For this review, take the finished solid that the model builds, in its own axes (mm). Face numbers are marked on the shaded views. A direction names the side the tool comes from. Coordinates: 2 decimals unless noted, no trailing zeros. Loops run counter-clockwise (first coordinate to the right, second up) from the corner with the lowest first, then second, coordinate; pieces in that order, holes last. Notation, with made-up numbers: (85.5, 34.5) - (126.5, 34.5) arc R20 cw to (126.5, 61.5) - close; hole circle Ø9 at (23, 58.25). An arc over 180 degrees is marked (long way). Answer as a JSON object with one key per item and string values. Group by question number.
Item 1: To check wall thickness, follow line 1 (Y direction, x = 3, z = -38.5); line 2 (Z direction, x = 1.7, y = -1.3); line 3 (Z direction, x = 2.35, y = 0.3). State the ranges of each line that lie inside material, in increasing order.
Item 2: Tool access review of the marked faces 1, 2 and 3: name each direction out of +Z, -Z, +X, -X, +Y, -Y from which nothing blocks a thin tool from reaching the whole face with its end or side.
Item 3: We need section B-B (x = 2.25). Give the boundary of the cut face in (y, z), then the cut area to 3 significant figures.
Item 4: We need section A-A (y = 0). Give the boundary of the cut face in (x, z).
Item 5: We need section C-C (z = -38). Give the boundary of the cut face in (x, y).
Item 6: Clearance check with flat-ended pins moving along their axes: pin 1 (3 mm diameter, centred on y = 0, z = -38.5, fed in from -X); pin 2 (3 mm diameter, centred on y = -1, z = -3.5, fed in from +X); pin 3 (0.6 mm diameter, centred on x = 3.5, y = -0.5, fed in from +Z); pin 4 (0.6 mm diameter, centred on x = 0.5, y = -1, fed in from -Z). State where each tip first meets the part, or that it passes through.
Item 7: We need section D-D (x = 0.55). Give the boundary of the cut face in (y, z), then the cut area to 3 significant figures.
from build123d import *

# Parameters (mm, degrees)
SKETCH1_R           = 1.65
BOSS_EXTRUDE1_DEPTH = 3
SKETCH3_W           = 11
SKETCH3_H           = 6
CUT_EXTRUDE2_DEPTH  = 1.2
SKETCH4_R           = 1.65
BOSS_EXTRUDE2_DEPTH = 1.2


with BuildPart() as part:
    # Sketch1 → Boss-Extrude1 (new body)
    with BuildSketch(Plane(origin=(0, 0, 0), x_dir=(0, 0, -1), z_dir=(1, 0, 0))):
        with BuildLine():
            Line((0, 3), (38.5, 3))
            ThreePointArc((38.5, 3), (41.5, 0), (38.5, -3))
            Line((38.5, -3), (0, -3))
            ThreePointArc((0, -3), (-3, 0), (0, 3))
        make_face()
        Circle(SKETCH1_R, mode=Mode.SUBTRACT)
        with Locations((38.5, 0)):
            Circle(SKETCH1_R, mode=Mode.SUBTRACT)
    extrude(amount=BOSS_EXTRUDE1_DEPTH)

    # Sketch3 → Cut-Extrude2 (cut)
    with BuildSketch(Plane.ZY):
        with Locations((-36, 0)):
            Rectangle(SKETCH3_W, SKETCH3_H)
    extrude(amount=-CUT_EXTRUDE2_DEPTH, mode=Mode.SUBTRACT)

    # Sketch4 → Boss-Extrude2 (add)
    with BuildSketch(Plane(origin=(3, 0, 0), x_dir=(0, 0, -1), z_dir=(1, 0, 0))):
        with BuildLine():
            Line((38.5, 3), (21.5, 3))
            Line((21.5, 3), (21.5, -3))
            Line((21.5, -3), (38.5, -3))
            ThreePointArc((38.5, -3), (41.5, 0), (38.5, 3))
        make_face()
        with Locations((38.5, 0)):
            Circle(SKETCH4_R, mode=Mode.SUBTRACT)
    extrude(amount=BOSS_EXTRUDE2_DEPTH)


solid = part.part
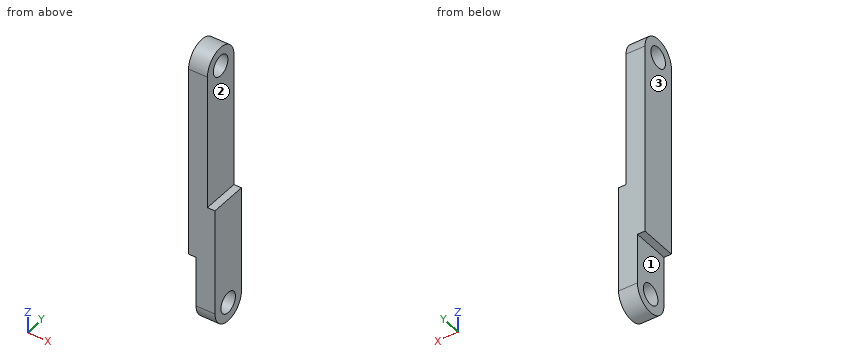
Check sheet entries:
{
 "1": {"line 1": "y = -3 to -1.65, 1.65 to 3", "line 2": "z = -41.2 to -39.52, -37.48 to -1.02, 1.02 to 2.7", "line 3": "z = -41.48 to -40.12, -36.88 to -1.62, 1.62 to 2.98"},
 "2": {"face 1": "-Z, -X, +Y, -Y", "face 2": "+Z, +X, +Y, -Y", "face 3": "+Z, -Z, -X, +Y, -Y"},
 "3": {"outline": "(-3, -38.5) arc R3 ccw to (3, -38.5) - (3, 0) arc R3 ccw to (-3, 0) - close; hole circle Ø3.3 at (0, -38.5); hole circle Ø3.3 at (0, 0)", "area": "242 mm2"},
 "4": {"outline": "(0, -30.5) - (1.2, -30.5) - (1.2, -36.85) - (4.2, -36.85) - (4.2, -21.5) - (3, -21.5) - (3, -1.65) - (0, -1.65) - close; (0, 1.65) - (3, 1.65) - (3, 3) - (0, 3) - close; (1.2, -41.5) - (4.2, -41.5) - (4.2, -40.15) - (1.2, -40.15) - close"},
 "5": {"outline": "(1.2, -3) - (4.2, -3) - (4.2, -1.57) - (1.2, -1.57) - close; (1.2, 1.57) - (4.2, 1.57) - (4.2, 3) - (1.2, 3) - close"},
 "6": {"pin 1": "passes through", "pin 2": "stops at x = 3", "pin 3": "stops at z = -21.5", "pin 4": "stops at z = -30.5"},
 "7": {"outline": "(-3, -30.5) - (3, -30.5) - (3, 0) arc R3 ccw to (-3, 0) - close; hole circle Ø3.3 at (0, 0)", "area": "189 mm2"}
}
